Verification items for the finished model (mm, model axes). A direction names the side the tool comes from. Round coordinates to 2 decimals unless told otherwise and drop trailing zeros. Loops run counter-clockwise (first coordinate to the right, second up) from the corner with the lowest first, then second, coordinate; pieces in that order, holes last. Notation, with made-up numbers: (10.25, 50) -> (28.25, 50) arc R18 ccw to (28.25, 67) -> close; hole circle Ø7 at (57, 56). An arc over 180 degrees is marked (long way). Write item = value, one per line. Start each with the question number.
```python
from build123d import *

# Parameters (mm, degrees)
BOSS_EXTRUDE2_DEPTH = 19.05
SKETCH3_R           = 39.496431486
SKETCH3_R_2         = 35.260007957
CUT_EXTRUDE2_DEPTH  = 1.778
SKETCH4_R           = 31.746180351
SKETCH4_R_2         = 28.068999156
CUT_EXTRUDE3_DEPTH  = 1.778
CUT_EXTRUDE4_START  = -1.778
SKETCH5_R           = 39.496431486
SKETCH5_R_2         = 35.260007957
CUT_EXTRUDE4_DEPTH  = 1.778
CUT_EXTRUDE5_START  = -1.778
SKETCH7_R           = 31.746180351
SKETCH7_R_2         = 28.068999156
CUT_EXTRUDE5_DEPTH  = 1.778
SKETCH8_R           = 15.24
BOSS_EXTRUDE3_DEPTH = 35.56


with BuildPart() as part:
    # Sketch2 → Boss-Extrude2 (new body)
    with BuildSketch(Plane.XY):
        with BuildLine():
            Line((20.429296249, -72.446914532), (20.429296249, -45.399816154))
            ThreePointArc((20.429296249, -45.399816154), (25.133677026, -34.04243628), (36.4910569, -29.338055504))
            Line((36.4910569, -29.338055504), (36.4910569, -20.532405534))
            ThreePointArc((36.4910569, -20.532405534), (20.935477727, -5.485511485), (0, 0))
            ThreePointArc((0, 0), (-20.935477727, -5.485511485), (-36.4910569, -20.532405534))
            Line((-36.4910569, -20.532405534), (-36.4910569, -29.338055504))
            ThreePointArc((-36.4910569, -29.338055504), (-25.133677026, -34.04243628), (-20.429296249, -45.399816154))
            Line((-20.429296249, -45.399816154), (-20.429296249, -72.446914532))
            ThreePointArc((-20.429296249, -72.446914532), (-12.360356233, -83.33771782), (0, -88.9))
            ThreePointArc((0, -88.9), (12.360356233, -83.33771782), (20.429296249, -72.446914532))
        make_face()
    extrude(amount=BOSS_EXTRUDE2_DEPTH)

    # Sketch3 → Cut-Extrude2 (cut)
    with BuildSketch(Plane.XY.offset(19.05)):
        with Locations((0, -44.45)):
            Circle(SKETCH3_R)
        with Locations((0, -44.45)):
            Circle(SKETCH3_R_2, mode=Mode.SUBTRACT)
    extrude(amount=-CUT_EXTRUDE2_DEPTH, mode=Mode.SUBTRACT)

    # Sketch4 → Cut-Extrude3 (cut)
    with BuildSketch(Plane.XY.offset(19.05)):
        with Locations((0, -44.45)):
            Circle(SKETCH4_R)
        with Locations((0, -44.45)):
            Circle(SKETCH4_R_2, mode=Mode.SUBTRACT)
    extrude(amount=-CUT_EXTRUDE3_DEPTH, mode=Mode.SUBTRACT)

    # Sketch5 → Cut-Extrude4 (cut)
    with BuildSketch(Plane(origin=(0, 0, 0), x_dir=(-1, 0, 0), z_dir=(0, 0, -1)).offset(CUT_EXTRUDE4_START)):
        with Locations((0, -44.45)):
            Circle(SKETCH5_R)
        with Locations((0, -44.45)):
            Circle(SKETCH5_R_2, mode=Mode.SUBTRACT)
    extrude(amount=CUT_EXTRUDE4_DEPTH, mode=Mode.SUBTRACT)

    # Sketch7 → Cut-Extrude5 (cut)
    with BuildSketch(Plane(origin=(0, 0, 0), x_dir=(-1, 0, 0), z_dir=(0, 0, -1)).offset(CUT_EXTRUDE5_START)):
        with Locations((0, -44.45)):
            Circle(SKETCH7_R)
        with Locations((0, -44.45)):
            Circle(SKETCH7_R_2, mode=Mode.SUBTRACT)
    extrude(amount=CUT_EXTRUDE5_DEPTH, mode=Mode.SUBTRACT)

    # Sketch8 → Boss-Extrude3 (add)
    with BuildSketch(Plane.XY.offset(19.05)):
        with Locations(Location((0, -62.23, 0), (0, 0, 206.225395775))):
            Circle(SKETCH8_R)
    extrude(amount=BOSS_EXTRUDE3_DEPTH)


solid = part.part
```
(1) Depth check by flat-ended pin: pin 1 Ø10.5 at (x, y) = (5, -19.5) entering from -Z; pin 2 Ø5.5 at (y, z) = (-58, 10.5) entering from +X; pin 3 Ø9.5 at (y, z) = (-54, 9.5) entering from -X; pin 4 Ø23.5 at (x, y) = (6.5, -22) entering from +Z. Enter the tip coordinate at first touch or a pass-through.
(2) Section check A-A on z = 10.5. Enter the section's corners in (x, y).
(3) Draft check along X on faces 1 (the flat face through (0, -8, 1.778)), 2 (the flat face through (0, -80, 17.272)), 3 (the cylindrical face through (-25.26, -33.92, 9.39)), 4 (the flat face through (20.429, -59, 9)). Enter one of: +X half, -X half, draft (parallel to the pull), parting line (faces both ways), or undercut.
(4) Section check D-D on y = -52. Enter the section's corners in (x, z), then the cut area to 3 significant figures.
(5) Section check C-C on x = -30. Enter the section's corners in (y, z), then the cut area to 3 significant figures.
(6) Access from +Z, -Z, +X, -X, +Y, -Y to the whole of each face (thin tool, end or side, straight path). Record for faces 5 (the cylindrical face through (-3.611, -47.424, 36.581)), 6 (the cylindrical face through (0.213, -83.946, 0.901)), 7 (the flat face through (-20.429, -59, 9)), 8 (the flat face through (-3, -12, 19.05)).
(7) Section check B-B on y = -62.23. Enter the section's corners in (x, z), then the cut area to 3 significant figures.
(8) Scan lines: line 1 (X direction, y = -61.5, z = 22); line 2 (Z direction, x = -5, y = -8.5); line 3 (Y direction, x = 24.5, z = 18). Record each from-to range of solid material in increasing order. Write a range as [from, to].
Computed values:
q1.pin_1 = 0
q1.pin_2 = 20.43
q1.pin_3 = -20.43
q1.pin_4 = 19.05
q2.outline = (-36.49, -29.34) arc R16.06 cw to (-20.43, -45.4) -> (-20.43, -72.45) arc R26.85 ccw to (0, -88.9) arc R26.85 ccw to (20.43, -72.45) -> (20.43, -45.4) arc R16.06 cw to (36.49, -29.34) -> (36.49, -20.53) arc R42.69 ccw to (-36.49, -20.53) -> close
q3.face_1 = undercut
q3.face_2 = undercut
q3.face_3 = -X half
q3.face_4 = +X half
q4.outline = (-20.43, 0) -> (20.43, 0) -> (20.43, 19.05) -> (11.3, 19.05) -> (11.3, 54.61) -> (-11.3, 54.61) -> (-11.3, 19.05) -> (-20.43, 19.05) -> close
q4.area = 1,580 mm²
q5.outline = (-30.71, 0) -> (-25.92, 0) -> (-25.92, 1.78) -> (-18.76, 1.78) -> (-18.76, 0) -> (-12.32, 0) -> (-12.32, 19.05) -> (-18.76, 19.05) -> (-18.76, 17.27) -> (-25.92, 17.27) -> (-25.92, 19.05) -> (-30.71, 19.05) -> close
q5.area = 325 mm²
q6.face_5 = +Z
q6.face_6 = -Z
q6.face_7 = +Z, -Z, -X, -Y
q6.face_8 = +Z, +X, -X, +Y
q7.outline = (-20.43, 0) -> (20.43, 0) -> (20.43, 19.05) -> (15.24, 19.05) -> (15.24, 54.61) -> (-15.24, 54.61) -> (-15.24, 19.05) -> (-20.43, 19.05) -> close
q7.area = 1,860 mm²
q8.line_1 = [-15.22, 15.22]
q8.line_2 = [1.78, 17.27]
q8.line_3 = [-34.71, -30.75], [-24.26, -19.09], [-13.47, -7.73]
